Part print with two shaded views. Sizes in mm from the minimum x, y, z corner. A direction names the side the tool comes from. Round coordinates to 2 decimals unless told otherwise and drop trailing zeros. Order: outer loops, then holes, each group sorted by start corner. A loop starts at its lowest first (then second) coordinate and runs counter-clockwise, first axis right, second up. Notation, with made-up numbers: M 79,-29.5 L 130,-29.5 A17 ccw 130,-25.5 Z; hole C 41,74.5 d6. An arc over 180 degrees is marked long. One line per question, with ' | ' between items. Start each with the question number.
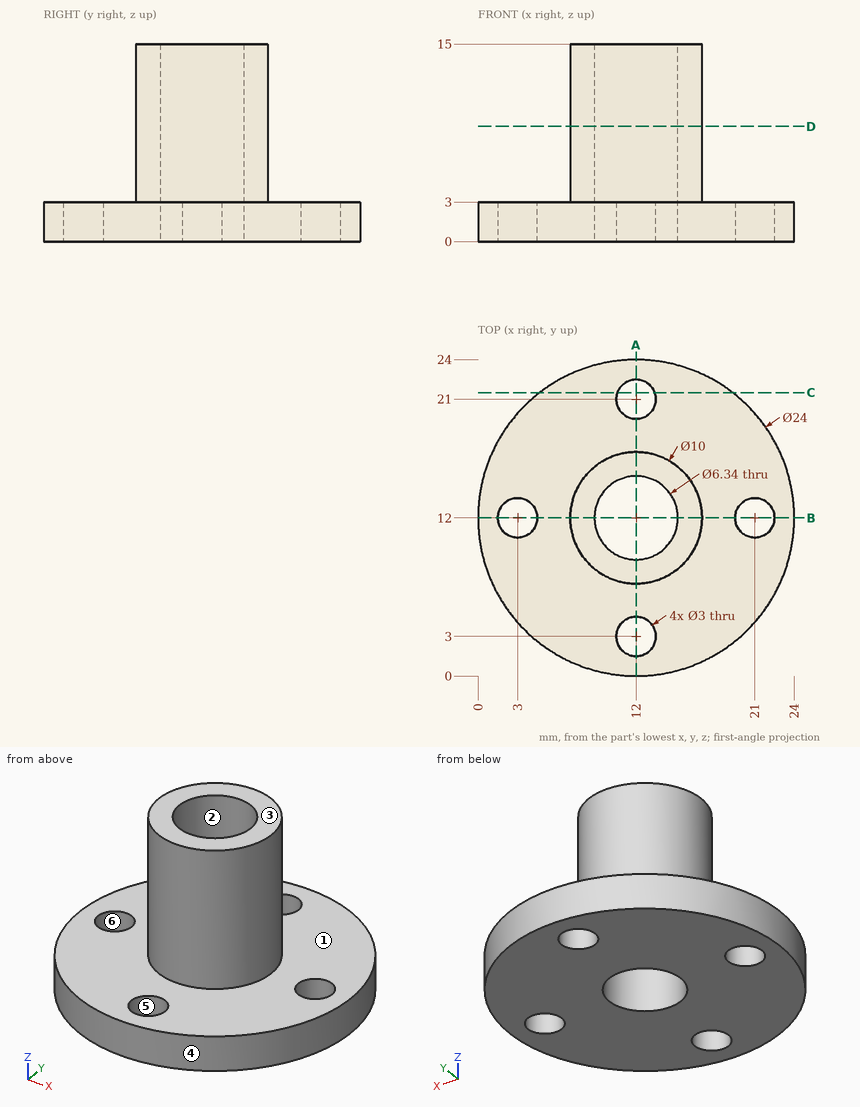
Item 1: Cut at C-C on y = 21.5. Write the cut outline in (x, z), then the cut area to 3 significant figures.
Item 2: Flat gauge pins, fed straight in: pin 1 (5 mm diameter, centred on y = 12, z = 11, fed in from +X); pin 2 (1.5 mm diameter, centred on x = 19, y = 20, fed in from +Z); pin 3 (5 mm diameter, centred on y = 7, z = 3, fed in from -X). Where does each tip first touch, or does it go through?
Item 3: Cut at A-A on x = 12. Write the cut outline in (y, z), then the cut area to 3 significant figures.
Item 4: Two-plate mould, pull along Y, no slides. Class the marked faces 3, 4, 5 and 6: +Y half, -Y half, draft (parallel to the pull), parting line (faces both ways), or undercut.
Item 5: Wall check: line 1 along Y through (x, z) = (12, 2.35); line 2 along Z through (x, y) = (5.75, 7); line 3 along X through (y, z) = (14, 4.25). Give the ranges that are in metal, low to high. Write a range as [from, to].
Item 6: Tool access for the marked faces 1 and 2: list every direction of +Z, -Z, +X, -X, +Y, -Y with a clear straight run to the whole face (end or side of a thin tool).
Item 7: Cut at D-D on z = 8.75. Write the cut outline in (x, y), then the cut area to 3 significant figures.
Results found:
1) outline: M 4.67,0 L 10.59,0 L 10.59,3 L 4.67,3 Z; M 13.41,0 L 19.33,0 L 19.33,3 L 13.41,3 Z | area: 35.5 mm^2
2) pin 1: stops at x = 17 | pin 2: stops at z = 3 | pin 3: stops at x = 0.26
3) outline: M 0,0 L 1.5,0 L 1.5,3 L 0,3 Z; M 4.5,0 L 8.83,0 L 8.83,15 L 7,15 L 7,3 L 4.5,3 Z; M 15.17,0 L 19.5,0 L 19.5,3 L 17,3 L 17,15 L 15.17,15 Z; M 22.5,0 L 24,0 L 24,3 L 22.5,3 Z | area: 78.9 mm^2
4) face 3: draft | face 4: parting line | face 5: undercut | face 6: undercut
5) line 1: y = [0, 1.5], [4.5, 8.83], [15.17, 19.5], [22.5, 24] | line 2: z = [0, 3] | line 3: x = [7.42, 9.54], [14.46, 16.58]
6) face 1: +Z | face 2: +Z, -Z
7) outline: C 12,12 d10; hole C 12,12 d6.34 | area: 47.0 mm^2
